Can you work these out from the model? Positions are in its coordinate system, mm. A direction names the side the tool comes from. Give positions to 0.01 mm unless a question says otherwise; leave off trailing zeros. Loops run counter-clockwise (first coordinate to the right, second up) from the corner with the lowest first, then second, coordinate; pieces in that order, holes last. Notation, with made-up numbers: (27.5, 50) - (65.5, 50) arc R7 cw to (65.5, 59) - close; hole circle Ø10 at (-11, 72). An arc over 180 degrees is marked (long way). Answer as a JSON object with one key per item and string values.
```python
from build123d import *

# Parameters (mm, degrees)
SKETCH1_R             = 4
BOSS_EXTRUDE1_DEPTH   = 19.05
SKETCH2_R             = 7.5
CUT_EXTRUDE1_DEPTH    = 8
M6X1_0_TAPPED_HOLE1_D = 5


with BuildPart() as part:
    # Sketch1 → Boss-Extrude1 (new body)
    with BuildSketch(Plane(origin=(0, 0, 0), x_dir=(1, 0, 0), z_dir=(0, 1, 0))):
        with BuildLine():
            Line((-43, -45), (43, -45))
            ThreePointArc((43, -45), (44.414213562, -44.414213562), (45, -43))
            Line((45, -43), (45, 43))
            ThreePointArc((45, 43), (44.414213562, 44.414213562), (43, 45))
            Line((43, 45), (-43, 45))
            ThreePointArc((-43, 45), (-44.414213562, 44.414213562), (-45, 43))
            Line((-45, 43), (-45, -43))
            ThreePointArc((-45, -43), (-44.414213562, -44.414213562), (-43, -45))
        make_face()
        with Locations((-32.5, 32.5)):
            Circle(SKETCH1_R, mode=Mode.SUBTRACT)
        with Locations((32.5, 32.5)):
            Circle(SKETCH1_R, mode=Mode.SUBTRACT)
        with Locations((32.5, -32.5)):
            Circle(SKETCH1_R, mode=Mode.SUBTRACT)
        with Locations((-32.5, -32.5)):
            Circle(SKETCH1_R, mode=Mode.SUBTRACT)
    extrude(amount=BOSS_EXTRUDE1_DEPTH)

    # Sketch2 → Cut-Extrude1 (cut)
    with BuildSketch(Plane(origin=(0, 19.05, 0), x_dir=(1, 0, 0), z_dir=(0, 1, 0))):
        with Locations((-32.5, -32.5)):
            Circle(SKETCH2_R)
        with Locations((32.5, -32.5)):
            Circle(SKETCH2_R)
        with Locations((32.5, 32.5)):
            Circle(SKETCH2_R)
        with Locations((-32.5, 32.5)):
            Circle(SKETCH2_R)
    extrude(amount=-CUT_EXTRUDE1_DEPTH, mode=Mode.SUBTRACT)

    # M6x1.0 Tapped Hole1 (through all)
    with Locations(Plane(origin=(0, 19.05, 0), x_dir=(1, 0, 0), z_dir=(0, 1, 0))):
        with Locations((-32.5, 0), (32.5, 0)):
            Hole(M6X1_0_TAPPED_HOLE1_D / 2)


solid = part.part
```
1) Imagine slicing it at A-A on y = 6.5. Write out the boundary of the cut face in (x, z).
Check sheet entries:
{"outline": "(-45, -43) arc R2 ccw to (-43, -45) - (43, -45) arc R2 ccw to (45, -43) - (45, 43) arc R2 ccw to (43, 45) - (-43, 45) arc R2 ccw to (-45, 43) - close; hole circle Ø8 at (-32.5, -32.5); hole circle Ø8 at (-32.5, 32.5); hole circle Ø5 at (-32.5, 0); hole circle Ø8 at (32.5, -32.5); hole circle Ø8 at (32.5, 32.5); hole circle Ø5 at (32.5, 0)"}
2) Imagine slicing it at B-B on x = 32.5. Write out the boundary of the cut face in (y, z), and give its area (3 significant figures).
Check sheet entries:
{"outline": "(0, -45) - (19.05, -45) - (19.05, -40) - (11.05, -40) - (11.05, -36.5) - (0, -36.5) - close; (0, -28.5) - (11.05, -28.5) - (11.05, -25) - (19.05, -25) - (19.05, -2.5) - (0, -2.5) - close; (0, 2.5) - (19.05, 2.5) - (19.05, 25) - (11.05, 25) - (11.05, 28.5) - (0, 28.5) - close; (0, 36.5) - (11.05, 36.5) - (11.05, 40) - (19.05, 40) - (19.05, 45) - (0, 45) - close", "area": "1,200 mm2"}
3) Imagine slicing it at D-D on y = 14.25. Write out the boundary of the cut face in (x, z), and give its area (3 significant figures).
Check sheet entries:
{"outline": "(-45, -43) arc R2 ccw to (-43, -45) - (43, -45) arc R2 ccw to (45, -43) - (45, 43) arc R2 ccw to (43, 45) - (-43, 45) arc R2 ccw to (-45, 43) - close; hole circle Ø15 at (-32.5, -32.5); hole circle Ø15 at (-32.5, 32.5); hole circle Ø5 at (-32.5, 0); hole circle Ø15 at (32.5, -32.5); hole circle Ø15 at (32.5, 32.5); hole circle Ø5 at (32.5, 0)", "area": "7,350 mm2"}
4) Imagine slicing it at C-C on z = 32.5. Write out the boundary of the cut face in (x, y), and give its area (3 significant figures).
Check sheet entries:
{"outline": "(-45, 0) - (-36.5, 0) - (-36.5, 11.05) - (-40, 11.05) - (-40, 19.05) - (-45, 19.05) - close; (-28.5, 0) - (28.5, 0) - (28.5, 11.05) - (25, 11.05) - (25, 19.05) - (-25, 19.05) - (-25, 11.05) - (-28.5, 11.05) - close; (36.5, 0) - (45, 0) - (45, 19.05) - (40, 19.05) - (40, 11.05) - (36.5, 11.05) - close", "area": "1,300 mm2"}
5) If we mould it in two halves opening along X, with no side actions, what happens to faces 1 (the flat face through (1, 9, -45)), 2 (the cylindrical face through (30.87, 15.11, 39.82)), 3 (the cylindrical face through (-44.43, 9.39, 44.4))? For each: released by +X, released by -X, zero draft, split by the parting line, or undercut.
Check sheet entries:
{"face 1": "zero draft", "face 2": "undercut", "face 3": "released by -X"}
6) Which directions (+Z, -Z, +X, -X, +Y, -Y) give clear straight access to the entire face, cutting with the end or side of a thin tool? Please do faces 4 (the flat face through (45, 9, 1)), 5 (the flat face through (-29, 11.05, 36)).
Check sheet entries:
{"face 4": "+Z, -Z, +X, +Y, -Y", "face 5": "+Y"}
7) I need wall thicknesses on L1, parallel to Z at x = 32.5, y = 15; L2, parallel to X at y = 3, z = 32.5; L3, parallel to X at y = 15.25, z = 32.5. Which ranges of each line are inside material? Lowest first, please.
Check sheet entries:
{"L1": "-45 to -40, -25 to -2.5, 2.5 to 25, 40 to 45", "L2": "-45 to -36.5, -28.5 to 28.5, 36.5 to 45", "L3": "-45 to -40, -25 to 25, 40 to 45"}
8) I'm going to push flat-ended pins straight in: P1, Ø4, axis at x = 32.5, z = 0, coming from the -Y side; P2, Ø12, axis at x = -32.5, z = 31.5, coming from the +Y side. Where does each tip first touch, or does it pass through?
Check sheet entries:
{"P1": "through", "P2": "y = 11.05"}
